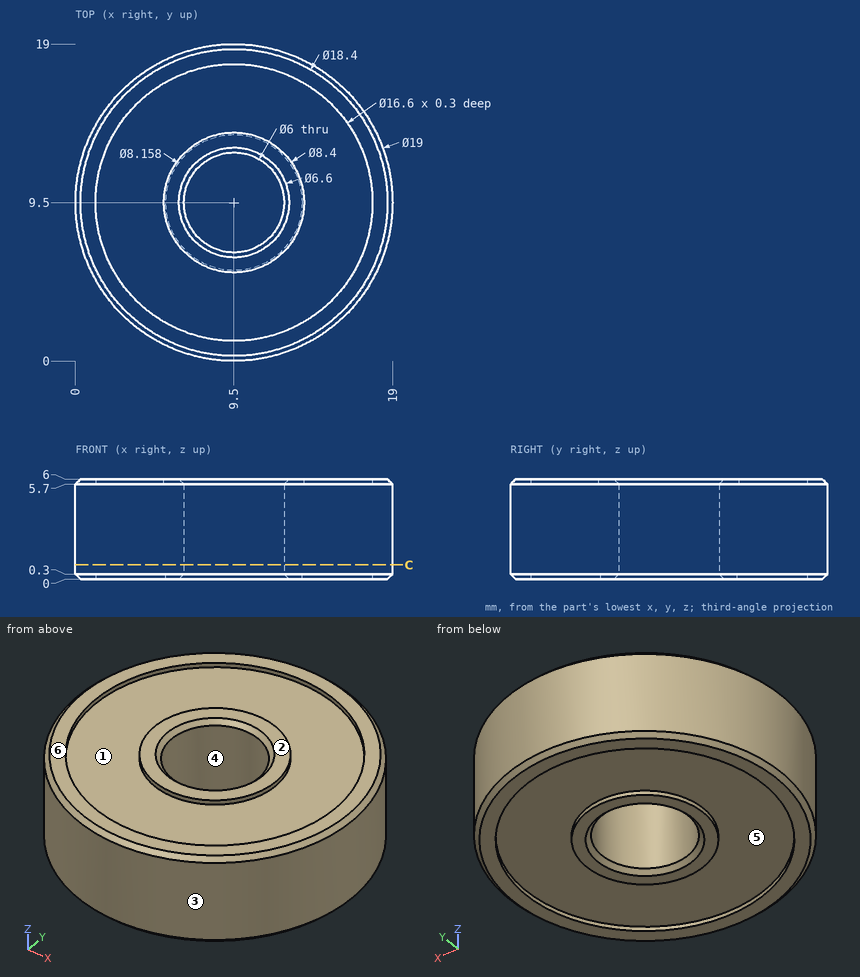
Can you work these out from the drawing? Everything is in mm from the part's minimum corner. A direction names the side the tool comes from. Coordinates: 2 decimals unless noted, no trailing zeros. Loops run counter-clockwise (first coordinate to the right, second up) from the corner with the lowest first, then second, coordinate; pieces in that order, holes last. Notation, with made-up numbers: M 38.25,5.25 L 79.25,5.25 A11 ccw 79.25,14.25 Z; hole C 80.25,20.5 d11. An arc over 180 degrees is marked long. Put each result on its own line as item: value. Start each with the question number.
(1) For the marked faces 1 and 2, which set-ups out of +Z, -Z, +X, -X, +Y, -Y let a thin tool reach every point of the face, with its end or its side?
(2) I need wall thicknesses on line 1 (Y direction, x = 9.5, z = 5.9); line 2 (X direction, y = 9.5, z = 5.95). Which ranges of each line are inside material? Lowest first, please. Write a range as from..to.
(3) Suppose I cut it at C-C on z = 0.85. Please give me the cut outline in (x, y).
(4) Will these pins go through, and if not, where does the flat tip stop? P1, Ø3, axis at y = 15, z = 4.5, coming from the +X side; P2, Ø2, axis at x = 4, z = 5.5, coming from the +Y side; P3, Ø3, axis at x = 7.5, z = 3, coming from the +Y side.
(5) Thinking about a two-plate mould opening in Y: for the marked faces 3, 4, 5 and 6, which applies, pulls with the +Y half, pulls with the -Y half, needs draft (parallel to the pull), parting line crosses it, or undercut?
Solutions:
1. face 1: +Z
1. face 2: +Z, +X, -X, +Y, -Y
2. line 1: y = 0.2..1.2, 5.3..6.3, 12.7..13.7, 17.8..18.8
2. line 2: x = 0.25..1.2, 5.3..6.25, 12.75..13.7, 17.8..18.75
3. outline: C 9.5,9.5 d19; hole C 9.5,9.5 d6
4. P1: stops at x = 18.12
4. P2: stops at y = 17.87
4. P3: stops at y = 18.99
5. face 3: parting line crosses it
5. face 4: undercut
5. face 5: undercut
5. face 6: needs draft
